```python
from build123d import *

# Parameters (mm, degrees)
BOSS_EXTRUDE1_DEPTH = 3
SKETCH3_R           = 2.5
SKETCH3_R_2         = 20
CUT_EXTRUDE1_DEPTH  = 10


with BuildPart() as part:
    # Sketch1 → Boss-Extrude1 (new body)
    with BuildSketch(Plane(origin=(0, 0, 0), x_dir=(1, 0, 0), z_dir=(0, 1, 0))):
        Polygon((-148.288384344, -111.309139144), (-148.288384344, -101.609139144), (-151.288384344, -101.609139144), (-151.288384344, -61.609139144), (-92.878384344, -61.609139144), (-92.878384344, -26.459139144), (-62.728384344, -26.459139144), (-62.728384344, -29.459139144), (-53.028384344, -29.459139144), (-53.028384344, -26.459139144), (-22.878384344, -26.459139144), (-22.878384344, -61.609139144), (35.531615656, -61.609139144), (35.531615656, -101.609139144), (32.531615656, -101.609139144), (32.531615656, -111.309139144), (35.531615656, -111.309139144), (35.531615656, -151.309139144), (-151.288384344, -151.309139144), (-151.288384344, -111.309139144), align=None)
    extrude(amount=BOSS_EXTRUDE1_DEPTH)

    # Sketch3 → Cut-Extrude1 (cut)
    with BuildSketch(Plane(origin=(0, 3, 0), x_dir=(1, 0, 0), z_dir=(0, 1, 0))):
        with Locations(Location((-77.878384344, -36.459139144, 0), (0, 0, 270))):
            Circle(SKETCH3_R)
        with Locations(Location((-37.878384344, -36.459139144, 0), (0, 0, 270))):
            Circle(SKETCH3_R)
        with Locations(Location((-37.878384344, -76.459139144, 0), (0, 0, 90))):
            Circle(SKETCH3_R)
        with Locations(Location((-77.878384344, -76.459139144, 0), (0, 0, 90))):
            Circle(SKETCH3_R)
        with Locations(Location((-57.878384344, -56.459139144, 0), (0, 0, 270))):
            Circle(SKETCH3_R_2)
    extrude(amount=-CUT_EXTRUDE1_DEPTH, mode=Mode.SUBTRACT)


solid = part.part
```
The model under review builds one solid part; all positions refer to its coordinate system, in mm. Give positions to 0.01 mm unless a question says otherwise; leave off trailing zeros. Loops run counter-clockwise (first coordinate to the right, second up) from the corner with the lowest first, then second, coordinate; pieces in that order, holes last. Notation, with made-up numbers: (53.25, 60.5) - (93.25, 60.5) arc R24 cw to (93.25, 90.5) - close; hole circle Ø6 at (73.5, 43.25). An arc over 180 degrees is marked (long way). Answer as a JSON object with one key per item and string values.
Q1. Insertion check: pin 1 (1.5 mm diameter, centred on x = 15, z = 131.5, fed in from -Y); pin 2 (0.9 mm diameter, centred on y = 1.5, z = 51, fed in from +X); pin 3 (0.9 mm diameter, centred on x = -58.5, y = 1, fed in from -Z); pin 4 (3 mm diameter, centred on x = -37.88, z = 76.46, fed in from -Y). Each pin has a flat end and moves straight along its axis. Give the tip position at first contact, or say it passes through.
Worked out:
{"pin 1": "stops at y = 0", "pin 2": "stops at x = -22.88", "pin 3": "stops at z = 29.46", "pin 4": "passes through"}
Q2. Add section B-B on x = -108. State the section outline as (y, z) points.
Worked out:
{"outline": "(0, 61.61) - (3, 61.61) - (3, 151.31) - (0, 151.31) - close"}
Q3. Mouldability with a two-part tool opening along X and no side actions: class faces 1 (the flat face through (-57, 0, 102)), 2 (the cylindrical face through (-75.66, 1.52, 75.31)) as +X half, -X half, draft (parallel to the pull), parting line (faces both ways), or undercut.
Worked out:
{"face 1": "draft", "face 2": "undercut"}
Q4. To check wall thickness, follow line 1 along X through (y, z) = (2, 34.5); line 2 along Z through (x, y) = (-94, 1.85); line 3 along X through (y, z) = (1.15, 61). State the ranges of each line that lie inside material, in increasing order.
Worked out:
{"line 1": "x = -92.88 to -79.43, -76.33 to -39.43, -36.33 to -22.88", "line 2": "z = 61.61 to 151.31", "line 3": "x = -92.88 to -77.36, -38.4 to -22.88"}
Q5. Add section A-A on y = 1.25. State the section outline as (x, z) points.
Worked out:
{"outline": "(-151.29, 61.61) - (-92.88, 61.61) - (-92.88, 26.46) - (-62.73, 26.46) - (-62.73, 29.46) - (-53.03, 29.46) - (-53.03, 26.46) - (-22.88, 26.46) - (-22.88, 61.61) - (35.53, 61.61) - (35.53, 101.61) - (32.53, 101.61) - (32.53, 111.31) - (35.53, 111.31) - (35.53, 151.31) - (-151.29, 151.31) - (-151.29, 111.31) - (-148.29, 111.31) - (-148.29, 101.61) - (-151.29, 101.61) - close; hole circle Ø5 at (-77.88, 36.46); hole circle Ø5 at (-77.88, 76.46); hole circle Ø40 at (-57.88, 56.46); hole circle Ø5 at (-37.88, 36.46); hole circle Ø5 at (-37.88, 76.46)"}
